from build123d import *

# Parameters (mm, degrees)
ESQUISSE1_R        = 5.5
ESQUISSE1_R_2      = 5
BOSS_EXTRU_1_DEPTH = 1
ESQUISSE4_R        = 5
BOSS_EXTRU_2_DEPTH = 19
ESQUISSE5_W        = 15
ESQUISSE5_H        = 8.000613173
BOSS_EXTRU_3_DEPTH = 2


with BuildPart() as part:
    # Esquisse1 → Boss.-Extru.1 (new body)
    with BuildSketch(Plane.XY):
        Circle(ESQUISSE1_R)
        Circle(ESQUISSE1_R_2, mode=Mode.SUBTRACT)
    extrude(amount=-BOSS_EXTRU_1_DEPTH)

    # Esquisse4 → Boss.-Extru.2 (add)
    with BuildSketch(Plane.XY):
        Circle(ESQUISSE4_R)
    extrude(amount=-BOSS_EXTRU_2_DEPTH)

    # Esquisse5 → Boss.-Extru.3 (add)
    with BuildSketch(Plane(origin=(0, 0, -19), x_dir=(-1, 0, 0), z_dir=(0, 0, -1))):
        with Locations((4.560754253, -0.044546246)):
            Rectangle(ESQUISSE5_W, ESQUISSE5_H)
    extrude(amount=BOSS_EXTRU_3_DEPTH)


solid = part.part
Part model, mm, in its own coordinate system. A direction names the side the tool comes from. Round coordinates to 2 decimals unless told otherwise and drop trailing zeros. Write each loop counter-clockwise with the first axis right and the second up, starting at its lowest first coordinate (ties: lowest second). Pieces come first, ordered by that corner, then holes. Notation, with made-up numbers: M 40.5,19 L 52.5,19 A9 cw 52.5,30 Z; hole C 49,-9 d6. An arc over 180 degrees is marked long. Return JSON: item names as keys, results as strings. Group by question number.
(1) Two-plate mould, pull along Z, no slides. Class faces 5 (the face through (-1.08, -4.88, -9.87)), 6 (the face through (-4, 3.956, -20)), 7 (the face through (-4, 0, -21)), 8 (the face through (1.6, -4.9, -1)): +Z half, -Z half, draft (parallel to the pull), parting line (faces both ways), or undercut.
(2) Saw through at A-A on y = 0. Write the cut outline in (x, z), then the cut area to 3 significant figures.
(3) Pin check, flat tips, straight feed: pin 1 Ø2 at (y, z) = (-1, -15) entering from +X; pin 2 Ø4 at (y, z) = (0, -10.5) entering from -X; pin 3 Ø3 at (y, z) = (4, -17) entering from +X; pin 4 Ø4 at (x, z) = (-10.5, -15.5) entering from -Y. Stop position of each tip, or through.
(4) Saw through at C-C on z = -5.25. Write the cut outline in (x, y).
(5) Saw through at B-B on x = 0. Write the cut outline in (y, z).
(6) Drill centre lines: probe 1 along Z at (x, y) = (3.75, -2.5); probe 2 along Z at (x, y) = (-9, -1); probe 3 along X at (y, z) = (-0.25, -2.75). Where is each one in solid material? Low to high.
(7) Saw through at D-D on x = -10.5. Write the cut outline in (y, z), then the cut area to 3 significant figures.
(8) Which spindle directions (+Z, -Z, +X, -X, +Y, -Y) get a long thin tool onto all of the face, cutting with end or side? Do faces 1 (the face through (2.939, 0, -20)), 2 (the face through (-1.19, -5.37, -0.49)), 3 (the face through (0, -4.4, -19)), 4 (the face through (0, 0, 0)). Say none if no direction does.
Returned:
{
 "1": {"face 5": "undercut", "face 6": "draft", "face 7": "-Z half", "face 8": "undercut"},
 "2": {"outline": "M -12.06,-21 L 2.94,-21 L 2.94,-19 L 5,-19 L 5,-1 L 5.5,-1 L 5.5,0 L -5.5,0 L -5.5,-1 L -5,-1 L -5,-19 L -12.06,-19 Z", "area": "221 mm²"},
 "3": {"pin 1": "x = 5", "pin 2": "x = -5", "pin 3": "x = 4.33", "pin 4": "through"},
 "4": {"outline": "C 0,0 d10"},
 "5": {"outline": "M -5.5,-1 L -5,-1 L -5,-19 L -4.04,-19 L -4.04,-21 L 3.96,-21 L 3.96,-19 L 5,-19 L 5,-1 L 5.5,-1 L 5.5,0 L -5.5,0 Z"},
 "6": {"probe 1": "-19 to 0", "probe 2": "-21 to -19", "probe 3": "-4.99 to 4.99"},
 "7": {"outline": "M -4.04,-21 L 3.96,-21 L 3.96,-19 L -4.04,-19 Z", "area": "16.0 mm²"},
 "8": {"face 1": "-Z, +X, +Y, -Y", "face 2": "+Z", "face 3": "-Z, +X, -X, -Y", "face 4": "+Z, +X, -X, +Y, -Y"}
}
